The model under review builds one solid part; all positions refer to its coordinate system, in mm. Face numbers are marked on the shaded views. A direction names the side the tool comes from. Round coordinates to 2 decimals unless told otherwise and drop trailing zeros. Order: outer loops, then holes, each group sorted by start corner. A loop starts at its lowest first (then second) coordinate and runs counter-clockwise, first axis right, second up. Notation, with made-up numbers: M 78,57.25 L 99,57.25 A11 ccw 99,65.25 Z; hole C 9,-4.5 d11. An arc over 180 degrees is marked long. Use a Markdown table: item, result. Add a question column.
1. Insertion check: P1, Ø12, axis at x = 15, z = 5.5, coming from the -Y side; P2, Ø0.5, axis at y = 10, z = 4.5, coming from the -X side; P3, Ø2, axis at y = 14, z = 1.5, coming from the -X side; P4, Ø9, axis at x = -2.5, y = 10.5, coming from the +Z side. Each pin has a flat end and moves straight along its axis. Give the tip position at first contact, or say it passes through.
2. For the marked faces 4, 5 and 6, list the 3-axis set-ups (+Z, -Z, +X, -X, +Y, -Y) from which the entire face can be reached by the end or side of a thin tool; tool diameter is ignored.
3. The part is to be moulded in two halves that separate along Z. For the marked faces 1, 2 and 3, say which applies: +Z half, -Z half, draft (parallel to the pull), parting line (faces both ways), or undercut.
4. Consider section C-C on z = -6. State the section outline as (x, y) points.
5. Consider section A-A on z = 0. Count the separate pieces of the cut face and the enclosed holes in it, then the cut area to 3 significant figures.
6. To check wall thickness, follow probe 1 along Y at (x, z) = (20, -7); probe 2 along Z at (x, y) = (30, 2.25); probe 3 along X at (y, z) = (2.5, 0). State the ranges of each line that lie inside material, in increasing order.
7. Consider section B-B on y = 5.75. State the section outline as (x, z) points, then the cut area to 3 significant figures.
8. Consider section D-D on x = 0. State the section outline as (y, z) points, then the cut area to 3 significant figures.
from build123d import *

# Parameters (mm, degrees)
SKETCH1_R           = 4
BOSS_EXTRUDE1_DEPTH = 20
CUT_EXTRUDE1_DEPTH  = 20
SKETCH3_R           = 5
CUT_EXTRUDE2_DEPTH  = 20
SKETCH3_3_R         = 9
CUT_EXTRUDE3_DEPTH  = 3


with BuildPart() as part:
    # Sketch1 → Boss-Extrude1 (new body)
    with BuildSketch(Plane(origin=(0, 0, 0), x_dir=(1, 0, 0), z_dir=(0, 1, 0))):
        with BuildLine():
            Line((-30, -10), (30, -10))
            ThreePointArc((30, -10), (40, 0), (30, 10))
            Line((30, 10), (-30, 10))
            ThreePointArc((-30, 10), (-40, 0), (-30, -10))
        make_face()
        with Locations(Location((-30, 0, 0), (0, 0, 270))):
            Circle(SKETCH1_R, mode=Mode.SUBTRACT)
        with Locations(Location((30, 0, 0), (0, 0, 270))):
            Circle(SKETCH1_R, mode=Mode.SUBTRACT)
    extrude(amount=BOSS_EXTRUDE1_DEPTH)

    # Sketch2 → Cut-Extrude1 (cut)
    with BuildSketch(Plane.XY.offset(10)):
        with BuildLine():
            Line((-40, 12.5), (-17, 12.5))
            ThreePointArc((-17, 12.5), (-15.585786438, 11.914213562), (-15, 10.5))
            Line((-15, 10.5), (-15, 9.5))
            ThreePointArc((-15, 9.5), (-15.585786438, 8.085786438), (-17, 7.5))
            Line((-17, 7.5), (-40, 7.5))
            Line((-40, 7.5), (-40, 12.5))
        make_face()
        with BuildLine():
            Line((40, 7.5), (40, 12.5))
            Line((40, 12.5), (17, 12.5))
            ThreePointArc((17, 12.5), (15.585786438, 11.914213562), (15, 10.5))
            Line((15, 10.5), (15, 9.5))
            ThreePointArc((15, 9.5), (15.585786438, 8.085786438), (17, 7.5))
            Line((17, 7.5), (40, 7.5))
        make_face()
    extrude(amount=-CUT_EXTRUDE1_DEPTH, mode=Mode.SUBTRACT)

    # Sketch3 → Cut-Extrude2 (cut)
    with BuildSketch(Plane.XY.offset(10)):
        with Locations((0, 10)):
            Circle(SKETCH3_R)
    extrude(amount=-CUT_EXTRUDE2_DEPTH, mode=Mode.SUBTRACT)

    # Sketch3_3 → Cut-Extrude3 (cut)
    with BuildSketch(Plane.XY.offset(10)):
        with Locations((0, 10)):
            Circle(SKETCH3_3_R)
    extrude(amount=-CUT_EXTRUDE3_DEPTH, mode=Mode.SUBTRACT)


solid = part.part
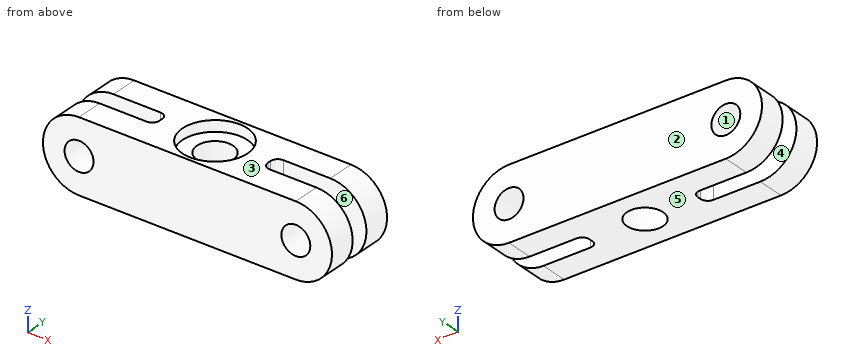
Answer block:
| question | item | result |
|---|---|---|
| 1 | P1 | y = 0 |
| 1 | P2 | x = -15 |
| 1 | P3 | x = -39.99 |
| 1 | P4 | z = 7 |
| 2 | face 4 | +Z, -Z, -X |
| 2 | face 5 | -Z, +X, -X, +Y, -Y |
| 2 | face 6 | +Z, -Z, +X |
| 3 | face 1 | undercut |
| 3 | face 2 | draft |
| 3 | face 3 | +Z half |
| 4 | outline | M -38,0 L 38,0 L 38,7.5 L 17,7.5 A2 cw 15,9.5 L 15,10.5 A2 cw 17,12.5 L 38,12.5 L 38,20 L -38,20 L -38,12.5 L -17,12.5 A2 cw -15,10.5 L -15,9.5 A2 cw -17,7.5 L -38,7.5 Z; hole C 0,10 d10 |
| 5 | separate pieces | 5 |
| 5 | enclosed holes | 1 |
| 5 | area | 1,030 mm^2 |
| 6 | probe 1 | 0 to 7.5, 12.5 to 20 |
| 6 | probe 2 | -10 to -4, 4 to 10 |
| 6 | probe 3 | -40 to -34, -26 to 26, 34 to 40 |
| 7 | outline | M -30,-10 L -2.63,-10 L -2.63,7 L -7.93,7 L -7.93,10 L -30,10 A10 ccw Z; M 2.63,-10 L 30,-10 A10 ccw 30,10 L 7.93,10 L 7.93,7 L 2.63,7 Z; hole C -30,0 d8; hole C 30,0 d8 |
| 7 | area | 1,280 mm^2 |
| 8 | outline | M 0,-10 L 5,-10 L 5,7 L 1,7 L 1,10 L 0,10 Z; M 15,-10 L 20,-10 L 20,10 L 19,10 L 19,7 L 15,7 Z |
| 8 | area | 176 mm^2 |
